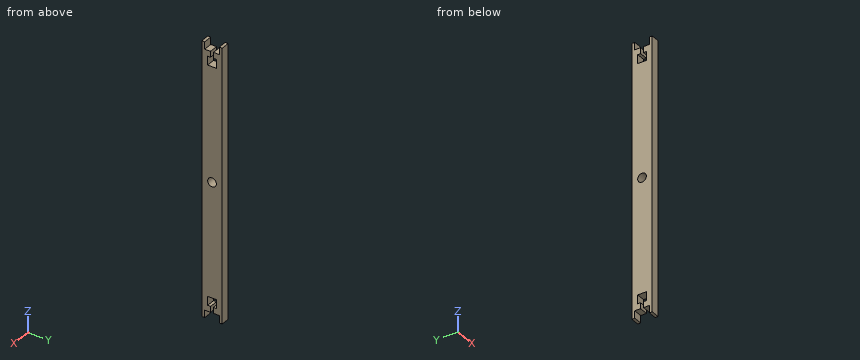
```python
from build123d import *

# Parameters (mm, degrees)
F1_DEPTH = 3
F2_R     = 1.5
F3_DEPTH = 3.001


with BuildPart() as f1:
    # F0 (on Right) → F1 (new body)
    with BuildSketch(Plane.YZ):
        Polygon((0, 93), (0, 0), (1, 0), (1, 2.5), (3, 2.5), (3, 4.5), (2, 4.5), (2, 7.5), (5, 7.5), (5, 4.5), (4, 4.5), (4, 2.5), (6, 2.5), (6, 0), (7, 0), (7, 93), (6, 93), (6, 90.5), (4, 90.5), (4, 88.5), (5, 88.5), (5, 85.5), (2, 85.5), (2, 88.5), (3, 88.5), (3, 90.5), (1, 90.5), (1, 93), align=None)
    extrude(amount=F1_DEPTH)

    # F2 (on face) → F3 (cut, through all)
    with BuildSketch(Plane.YZ.offset(3)):
        with Locations((3.5, 46.5)):
            Circle(F2_R)
    extrude(amount=-F3_DEPTH, mode=Mode.SUBTRACT)


solid = f1.part
```
The model under review builds one solid part; all positions refer to its coordinate system, in mm. Round coordinates to 2 decimals unless told otherwise and drop trailing zeros. Order: outer loops, then holes, each group sorted by start corner. A loop starts at its lowest first (then second) coordinate and runs counter-clockwise, first axis right, second up.
Item 1: For pin 1 (0.8 mm diameter, centred on x = 1.5, y = 4.5, fed in from -Z); pin 2 (0.8 mm diameter, centred on x = 2, y = 4.5, fed in from +Z), all flat-tipped, find the tip position at first contact; note any pin that passes through.
Working result:
pin 1: stops at z = 2.5
pin 2: stops at z = 90.5
Item 2: To check wall thickness, follow probe 1 along Y at (x, z) = (0.9, 5.5); probe 2 along Z at (x, y) = (2.4, 3.5); probe 3 along Z at (x, y) = (2.9, 2.25). State the ranges of each line that lie inside material, in increasing order.
Working result:
probe 1: y = 0 to 2, 5 to 7
probe 2: z = 7.5 to 45, 48 to 85.5
probe 3: z = 2.5 to 4.5, 7.5 to 45.67, 47.33 to 85.5, 88.5 to 90.5
Item 3: Add section A-A, the plane z = 46.5. State the section outline as (x, y) points, and give its area (3 significant figures).
Working result:
outline: (0, 0) - (3, 0) - (3, 2) - (0, 2) - close; (0, 5) - (3, 5) - (3, 7) - (0, 7) - close
area: 12.0 mm2
